CAD build for the part. Positions are in the model's coordinates, mm. Face numbers are marked on the shaded views. A direction names the side the tool comes from. Coordinates: 2 decimals unless noted, no trailing zeros. Write each loop counter-clockwise with the first axis right and the second up, starting at its lowest first coordinate (ties: lowest second). Pieces come first, ordered by that corner, then holes.
```python
from build123d import *

# Parameters (mm, degrees)
F0_W            = 210
F0_H            = 225
F1_DEPTH        = 25
F3_DEPTH        = 95
F5_DEPTH        = 10
F5_DEPTH_BACK   = 127
F7_DEPTH        = 10
F7_DEPTH_BACK   = 127
F8_W            = 60
F8_H            = 60
F9_DEPTH        = 10
F10_R           = 10
F12_DEPTH       = 20
F14_D           = 15
F14_CBORE_D     = 30
F14_CBORE_DEPTH = 10
F15_T1_DEPTH    = 20
F15_T6_DEPTH    = 80.7094158862
F15_S7_R        = 40
F15_T8_DEPTH    = 42
F15_T12_DEPTH   = 79.5275350517
F15_S13_R       = 40
F15_T14_DEPTH   = 42
F15_T18_DEPTH   = 82.0757730237
F15_S19_R       = 37.5
F15_T20_DEPTH   = 43
F16_R           = 19.5
F17_DEPTH       = 235.001
F18_R           = 19.5
F19_DEPTH       = 220.001


# Not quite as in the source:
# - a fillet or chamfer that OpenCascade refuses, or shapes differently, is made with other operations: its cross-section is extruded or revolved along the edge and cut away or added


with BuildPart() as f1:
    # F0 (on Top) → F1 (new body)
    with BuildSketch(Plane.XY):
        Rectangle(F0_W, F0_H)
    extrude(amount=F1_DEPTH)

    # F2 (on face) → F3 (join)
    with BuildSketch(Plane.XY.offset(25)):
        with BuildLine():
            Line((105, 48.5), (105, 63.5))
            Line((105, 63.5), (25, 63.5))
            ThreePointArc((25, 63.5), (-3.1177490061, -4.3822509939), (-71, -32.5))
            Line((-71, -32.5), (-71, -112.5))
            Line((-71, -112.5), (-56, -112.5))
            Line((-56, -112.5), (-56, -46.4818166789))
            ThreePointArc((-56, -46.4818166789), (7.4888527117, -14.9888527117), (38.9818166789, 48.5))
            Line((38.9818166789, 48.5), (105, 48.5))
        make_face()
    extrude(amount=F3_DEPTH)

    # F4 (on face) → F5 (join, two sides)
    with BuildSketch(Plane.XZ.offset(112.5)) as f5_sk:
        with BuildLine():
            ThreePointArc((-56, 83.2576538583), (-34.4526249034, 96.2829175487), (-26, 120))
            ThreePointArc((-26, 120), (-87.2170824513, 149.0473750966), (-71, 83.2576538583))
            Line((-71, 83.2576538583), (-71, 120))
            Line((-71, 120), (-56, 120))
            Line((-56, 120), (-56, 83.2576538583))
        make_face()
        with BuildLine():
            Line((-71, 120), (-71, 83.2576538583))
            ThreePointArc((-71, 83.2576538583), (-63.5, 82.5), (-56, 83.2576538583))
            Line((-56, 83.2576538583), (-56, 120))
            Line((-56, 120), (-71, 120))
        make_face()
    extrude(amount=F5_DEPTH)
    extrude(f5_sk.sketch, amount=-F5_DEPTH_BACK)

    # F6 (on face) → F7 (join, two sides)
    with BuildSketch(Plane.YZ.offset(105)) as f7_sk:
        with BuildLine():
            Line((48.5, 120), (48.5, 80.7094158862))
            ThreePointArc((48.5, 80.7094158862), (56, 80), (63.5, 80.7094158862))
            Line((63.5, 80.7094158862), (63.5, 120))
            Line((63.5, 120), (48.5, 120))
        make_face()
        with BuildLine():
            ThreePointArc((63.5, 80.7094158862), (86.8220700148, 94.504902432), (96, 120))
            ThreePointArc((96, 120), (30.504902432, 150.8220700148), (48.5, 80.7094158862))
            Line((48.5, 80.7094158862), (48.5, 120))
            Line((48.5, 120), (63.5, 120))
            Line((63.5, 120), (63.5, 80.7094158862))
        make_face()
    extrude(amount=F7_DEPTH)
    extrude(f7_sk.sketch, amount=-F7_DEPTH_BACK)

    # F8 (on face) → F9 (join)
    with BuildSketch(Plane.XY.offset(25)):
        with Locations((75, -82.5)):
            Rectangle(F8_W, F8_H)
    extrude(amount=F9_DEPTH)

    # F10
    f10_edges = [f1.edges().sort_by_distance(p)[0] for p in [
        (45, -52.5, 30),
    ]]
    fillet(f10_edges, radius=F10_R)

    # F11 (on face) → F12 (cut)
    with BuildSketch(Plane.XY.offset(25)):
        with BuildLine():
            ThreePointArc((46.5755076536, 39.5), (13.8528137424, -21.3528137424), (-47, -54.0755076536))
            Line((-47, -54.0755076536), (-47, -103.5))
            Line((-47, -103.5), (36, -103.5))
            Line((36, -103.5), (36, -62.5))
            ThreePointArc((36, -62.5), (41.5649711575, -49.0649711575), (55, -43.5))
            Line((55, -43.5), (96, -43.5))
            Line((96, -43.5), (96, 39.5))
            Line((96, 39.5), (46.5755076536, 39.5))
        make_face()
    extrude(amount=-F12_DEPTH, mode=Mode.SUBTRACT)

    # F14 (through all)
    with Locations(Plane.XY.offset(35)):
        with Locations((75, -82.5)):
            CounterBoreHole(F14_D / 2, F14_CBORE_D / 2, F14_CBORE_DEPTH)

    # F15: fillet of radius 10 on 8 edges, made by hand

    # F15_s2 → F15_t1 (join)
    with BuildSketch(Plane.XY.offset(5)):
        with BuildLine():
            ThreePointArc((-39.6153846154, -52.3231665823), (-44.9420981533, -55.8986609284), (-47, -61.9750971309))
            Line((-47, -61.9750971309), (-47, -54.0755076536))
            ThreePointArc((-47, -54.0755076536), (-43.2938349797, -53.257733876), (-39.6153846154, -52.3231665823))
        make_face()
        with BuildLine():
            ThreePointArc((44.8231665823, 32.1153846154), (48.3986609284, 37.4420981533), (54.4750971309, 39.5))
            Line((54.4750971309, 39.5), (46.5755076536, 39.5))
            ThreePointArc((46.5755076536, 39.5), (45.757733876, 35.7938349797), (44.8231665823, 32.1153846154))
        make_face()
        with BuildLine():
            ThreePointArc((96, 29.5), (93.0710678119, 36.5710678119), (86, 39.5))
            Line((86, 39.5), (96, 39.5))
            Line((96, 39.5), (96, 29.5))
        make_face()
        with BuildLine():
            ThreePointArc((86, -43.5), (93.0710678119, -40.5710678119), (96, -33.5))
            Line((96, -33.5), (96, -43.5))
            Line((96, -43.5), (86, -43.5))
        make_face()
        with BuildLine():
            ThreePointArc((-47, -93.5), (-44.0710678119, -100.5710678119), (-37, -103.5))
            Line((-37, -103.5), (-47, -103.5))
            Line((-47, -103.5), (-47, -93.5))
        make_face()
    extrude(amount=F15_T1_DEPTH)


with BuildPart() as f15_tool4:
    # F15_s5 → F15_t6 (new body)
    with BuildSketch(Plane.XY.offset(25)):
        with BuildLine():
            ThreePointArc((105, 53.5), (102.0710678119, 60.5710678119), (95, 63.5))
            Line((95, 63.5), (105, 63.5))
            Line((105, 63.5), (105, 53.5))
        make_face()
    extrude(amount=F15_T6_DEPTH)

    # F15_s7 → F15_t8 (cut, symmetric)
    with BuildSketch(Plane.YZ.offset(100)):
        with Locations((56, 120)):
            Circle(F15_S7_R)
    extrude(amount=F15_T8_DEPTH, both=True, mode=Mode.SUBTRACT)


with BuildPart() as f1_1:
    add(f1.part)

    # F15_t3: cut F15_tool4
    add(f15_tool4.part, mode=Mode.SUBTRACT)


with BuildPart() as f15_tool10:
    # F15_s11 → F15_t12 (new body)
    with BuildSketch(Plane.XY.offset(25)):
        with BuildLine():
            ThreePointArc((34.5272476662, 63.5), (27.7979818171, 60.8970927486), (24.571846943, 54.4433962264))
            ThreePointArc((24.571846943, 54.4433962264), (24.8929019962, 58.9666406785), (25, 63.5))
            Line((25, 63.5), (34.5272476662, 63.5))
        make_face()
    extrude(amount=F15_T12_DEPTH)

    # F15_s13 → F15_t14 (cut, symmetric)
    with BuildSketch(Plane.YZ.offset(29.5)):
        with Locations((56, 120)):
            Circle(F15_S13_R)
    extrude(amount=F15_T14_DEPTH, both=True, mode=Mode.SUBTRACT)


with BuildPart() as f1_2:
    add(f1_1.part)

    # F15_t9: cut F15_tool10
    add(f15_tool10.part, mode=Mode.SUBTRACT)


with BuildPart() as f15_tool16:
    # F15_s17 → F15_t18 (new body)
    with BuildSketch(Plane.XY.offset(25)):
        with BuildLine():
            ThreePointArc((-71, -42.0272476662), (-68.3970927486, -35.2979818171), (-61.9433962264, -32.071846943))
            ThreePointArc((-61.9433962264, -32.071846943), (-66.4666406785, -32.3929019962), (-71, -32.5))
            Line((-71, -32.5), (-71, -42.0272476662))
        make_face()
    extrude(amount=F15_T18_DEPTH)

    # F15_s19 → F15_t20 (cut, symmetric)
    with BuildSketch(Plane.XZ.offset(37)):
        with Locations((-63.5, 120)):
            Circle(F15_S19_R)
    extrude(amount=F15_T20_DEPTH, both=True, mode=Mode.SUBTRACT)


with BuildPart() as f1_3:
    add(f1_2.part)

    # F15_t15: cut F15_tool16
    add(f15_tool16.part, mode=Mode.SUBTRACT)

    # F16 (on face) → F17 (cut, through all)
    with BuildSketch(Plane.XZ.offset(122.5)):
        with Locations((-63.5, 120)):
            Circle(F16_R)
    extrude(amount=-F17_DEPTH, mode=Mode.SUBTRACT)

    # F18 (on face) → F19 (cut, through all)
    with BuildSketch(Plane.YZ.offset(115)):
        with Locations((56, 120)):
            Circle(F18_R)
    extrude(amount=-F19_DEPTH, mode=Mode.SUBTRACT)


solid = f1_3.part
```
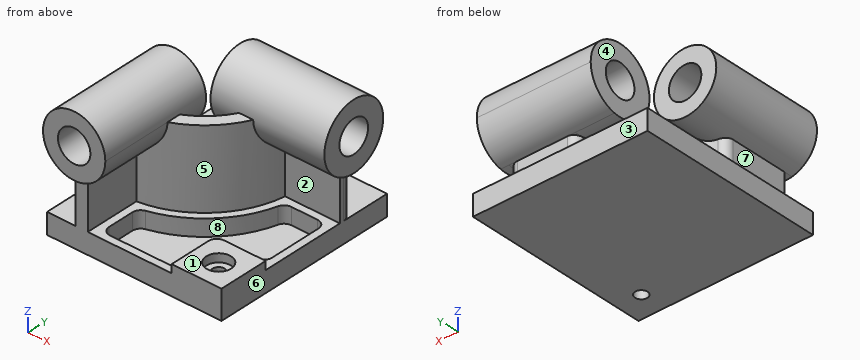
Item 1: Saw through at A-A, the plane y = -82.5. Write the cut outline in (x, z), and give its area (3 significant figures).
Item 2: Which spindle directions (+Z, -Z, +X, -X, +Y, -Y) get a long thin tool onto all of the face, cutting with end or side? Do the marked faces 4, 5, 6, 7 and 8. Say none if no direction does.
Item 3: Saw through at D-D, the plane x = -52. Write the cut outline in (y, z).
Item 4: Wall check: line 1 along Y through (x, z) = (75, 13); line 2 along Y through (x, z) = (75, 31); line 3 along X through (y, z) = (-78.5, 11). Give the ranges that are in metal, low to high.
Item 5: Saw through at C-C, the plane z = 124.5. Write the cut outline in (x, y), and give its area (3 significant figures).
Item 6: Flat gauge pins, fed straight in: pin 1 Ø6 at (x, z) = (72, 17) entering from -Y; pin 2 Ø12 at (x, y) = (32.5, -75.5) entering from +Z; pin 3 Ø10 at (y, z) = (-85.5, 16) entering from +X. Where does each tip first touch, or does it go through?
Item 7: Saw through at B-B, the plane x = 75. Write the cut outline in (y, z).
Item 8: Two-plate mould, pull along Z, no slides. Class the marked faces 1, 2 and 3: +Z half, -Z half, draft (parallel to the pull), parting line (faces both ways), or undercut.
Working result:
1. outline: (-105, 0) - (67.5, 0) - (67.5, 25) - (60, 25) - (60, 35) - (45, 35) - (45, 25) - (36, 25) - (36, 5) - (-47, 5) - (-47, 25) - (-56, 25) - (-56, 83.26) arc R37.5 ccw (long way) to (-71, 83.26) - (-71, 25) - (-105, 25) - close; (82.5, 0) - (105, 0) - (105, 35) - (90, 35) - (90, 25) - (82.5, 25) - close; hole circle Ø39 at (-63.5, 120)
1. area: 7,600 mm2
2. face 4: +Z, -X, +Y
2. face 5: +X, -Y
2. face 6: -Z, +X, +Y, -Y
2. face 7: -X, +Y, -Y
2. face 8: none
3. outline: (-122.5, 84.31) - (-45.86, 84.31) - (-45.86, 25) - (-112.5, 25) - (-112.5, 0) - (112.5, 0) - (112.5, 25) - (-30.6, 25) - (-30.6, 84.31) - (14.5, 84.31) - (14.5, 104.25) - (-122.5, 104.25) - close; (-122.5, 135.75) - (14.5, 135.75) - (14.5, 155.69) - (-122.5, 155.69) - close
4. line 1: y = -112.5 to -90, -75 to -43.5, 39.5 to 112.5
4. line 2: y = -112.5 to -97.5, -67.5 to -52.5, 48.5 to 63.5
4. line 3: x = -105 to -47, 36 to 68.66, 81.34 to 105
5. outline: (-100.73, -122.5) - (-82.47, -122.5) - (-82.47, 14.5) - (-100.73, 14.5) - close; (-44.53, -122.5) - (-26.27, -122.5) - (-26.27, 14.5) - (-44.53, 14.5) - close; (-22, 16.25) - (115, 16.25) - (115, 37.03) - (-22, 37.03) - close; (-22, 74.97) - (115, 74.97) - (115, 95.75) - (-22, 95.75) - close
5. area: 10,700 mm2
6. pin 1: stops at y = -112.5
6. pin 2: stops at z = 25
6. pin 3: stops at x = 105
7. outline: (-112.5, 0) - (-90, 0) - (-90, 25) - (-97.5, 25) - (-97.5, 35) - (-112.5, 35) - close; (-75, 0) - (112.5, 0) - (112.5, 25) - (63.5, 25) - (63.5, 80.71) arc R40 ccw (long way) to (48.5, 80.71) - (48.5, 25) - (39.5, 25) - (39.5, 5) - (-43.5, 5) - (-43.5, 25) - (-52.5, 25) - (-52.5, 35) - (-67.5, 35) - (-67.5, 25) - (-75, 25) - close; hole circle Ø39 at (56, 120)
8. face 1: +Z half
8. face 2: undercut
8. face 3: draft
